from build123d import *
from build123d.topology import SkipClean

# Parameters (mm, degrees)
SKETCH1_R            = 1.5
BOSS_EXTRUDE1_DEPTH  = 2
BOSS_EXTRUDE2_START  = 3
SKETCH2_R            = 2.5
SKETCH2_R_2          = 1.5
BOSS_EXTRUDE2_DEPTH  = 3
CUT_EXTRUDE1_REACH   = 126.021
SKETCH3_R            = 2.5
LPATTERN1_COUNT      = 3
LPATTERN1_PITCH      = 40.75
LPATTERN1_COUNT_DIR2 = 3
LPATTERN1_PITCH_DIR2 = 10
SKETCH4_W            = 2
SKETCH4_H            = 29.25
BOSS_EXTRUDE3_DEPTH  = 2


with BuildPart() as part:
    # Sketch1 → Boss-Extrude1 (new body)
    with BuildSketch(Plane(origin=(0, 0, 0), x_dir=(1, 0, 0), z_dir=(0, 1, 0))):
        Polygon((-112.25, 0), (0, 0), (0, 33.5), (-16, 33.5), (-16, 52.5), (-112.25, 52.5), align=None)
        with Locations(Location((-47.25, 49, 0), (0, 0, 270))):
            Circle(SKETCH1_R, mode=Mode.SUBTRACT)
        with Locations(Location((-108.75, 37.5, 0), (0, 0, 270))):
            Circle(SKETCH1_R, mode=Mode.SUBTRACT)
    extrude(amount=BOSS_EXTRUDE1_DEPTH)

    # Sketch2 → Boss-Extrude2 (add)
    with SkipClean():  # the faces are left unmerged after this step: merging them gives an invalid solid
        with BuildSketch(Plane(origin=(0, 0, 0), x_dir=(-1, 0, 0), z_dir=(0, -1, 0)).offset(BOSS_EXTRUDE2_START)):
            with Locations(Location((108.75, 37.5, 0), (0, 0, 90))):
                Circle(SKETCH2_R)
            with Locations(Location((108.75, 37.5, 0), (0, 0, 90))):
                Circle(SKETCH2_R_2, mode=Mode.SUBTRACT)
        extrude(amount=-BOSS_EXTRUDE2_DEPTH)

    # Sketch3 → Cut-Extrude1 (cut, up to next)
    with BuildSketch(Plane(origin=(0, 2, 0), x_dir=(1, 0, 0), z_dir=(0, 1, 0)), mode=Mode.PRIVATE) as cut_extrude1_sk1:
        with Locations(Location((-3.75, 26.75, 0), (0, 0, 270))):
            Circle(SKETCH3_R)
    cut_extrude1_tool1 = extrude(cut_extrude1_sk1.sketch, amount=-CUT_EXTRUDE1_REACH, mode=Mode.PRIVATE) & part.part
    # Sketch3 → Cut-Extrude1 (cut, up to next)
    with BuildSketch(Plane(origin=(0, 2, 0), x_dir=(1, 0, 0), z_dir=(0, 1, 0)), mode=Mode.PRIVATE) as cut_extrude1_sk2:
        with BuildLine():
            Line((-37.25, 29.25), (-11.25, 29.25))
            ThreePointArc((-11.25, 29.25), (-8.75, 26.75), (-11.25, 24.25))
            Line((-11.25, 24.25), (-37.25, 24.25))
            ThreePointArc((-37.25, 24.25), (-39.75, 26.75), (-37.25, 29.25))
        make_face()
    cut_extrude1_tool2 = extrude(cut_extrude1_sk2.sketch, amount=-CUT_EXTRUDE1_REACH, mode=Mode.PRIVATE) & part.part
    cut_extrude1_1 = cut_extrude1_tool1.solids().sort_by_distance((-3.75, 2, -26.75))[0]
    add(cut_extrude1_1, mode=Mode.SUBTRACT)
    cut_extrude1_2 = cut_extrude1_tool2.solids().sort_by_distance((-24.25, 2, -26.75))[0]
    add(cut_extrude1_2, mode=Mode.SUBTRACT)
    cut_extrude1 = cut_extrude1_1 + cut_extrude1_2  # Cut-Extrude1 as one shape, for the pattern or mirror that repeats it

    # LPattern1: Cut-Extrude1 3 × 3
    with SkipClean():  # the faces are left unmerged after this step: merging them gives an invalid solid
        with Locations(*[(-i * LPATTERN1_PITCH, 0, j * LPATTERN1_PITCH_DIR2) for i in range(LPATTERN1_COUNT) for j in range(LPATTERN1_COUNT_DIR2) if (i, j) != (0, 0)]):
            add(cut_extrude1, mode=Mode.SUBTRACT)

    # Sketch4 → Boss-Extrude3 (add)
    with SkipClean():  # the faces are left unmerged after this step: merging them gives an invalid solid
        with BuildSketch(Plane(origin=(0, 2, 0), x_dir=(1, 0, 0), z_dir=(0, 1, 0))):
            with Locations((-111.25, 14.625)):
                Rectangle(SKETCH4_W, SKETCH4_H)
        extrude(amount=-BOSS_EXTRUDE3_DEPTH)


solid = part.part
Can you work these out from the model? Positions are in its coordinate system, mm. A direction names the side the tool comes from. Round coordinates to 2 decimals unless told otherwise and drop trailing zeros. Write each loop counter-clockwise with the first axis right and the second up, starting at its lowest first coordinate (ties: lowest second). Pieces come first, ordered by that corner, then holes. Notation, with made-up numbers: (84, 80.5) -> (88, 80.5) arc R20 cw to (88, 113.5) -> close; hole circle Ø6 at (83.25, -1). An arc over 180 degrees is marked (long way). One line per question, with ' | ' between items. Start each with the question number.
1) Suppose I cut it at B-B on z = -26.75. Write out the boundary of the cut face in (x, y).
2) I'm going to push flat-ended pins straight in: P1, Ø6.5, axis at x = -44.5, z = -26.75, coming from the -Y side; P2, Ø2, axis at y = -2, z = -12, coming from the +X side; P3, Ø2, axis at y = 1, z = -43, coming from the +X side. Where does each tip first touch, or does it pass through?
3) Suppose I cut it at C-C on y = -1.35. Write out the boundary of the cut face in (x, z), then the cut area to 3 significant figures.
4) Suppose I cut it at A-A on x = -85.25. Write out the boundary of the cut face in (y, z), then the cut area to 3 significant figures.
5) On a 3-axis mill with a long thin cutter (end or side, diameter ignored), from which of +Z, -Z, +X, -X, +Y, -Y can I reach the whole of each face in a straight line? I mean faces 1 (the cylindrical face through (-90.25, 1.01, -26.8)), 2 (the flat face through (0, 1, -17)). Say none if no direction works.
6) If we mould it in two halves opening along X, with no side actions, what happens to faces 3 (the flat face through (-102, 1, -19.25)), 4 (the flat face through (-65, 1, -29.25)), 5 (the flat face through (-112.25, 1, -27)), 6 (the flat face through (-110, -3, -39))? For each: released by +X, released by -X, zero draft, split by the parting line, or undercut.
7) I need wall thicknesses on line 1 (Z direction, x = -20, y = 1.05); line 2 (X direction, y = 0.5, z = -49); line 3 (Y direction, x = -69.5, z = -42.5). Which ranges of each line are inside material? Lowest first, please. Write a range as [from, to].
8) Suppose I cut it at D-D on z = -17. Write out the boundary of the cut face in (x, y).
Return value:
1) outline: (-112.25, 0) -> (-110.25, 0) -> (-110.25, 2) -> (-112.25, 2) -> close; (-90.25, 0) -> (-87.75, 0) -> (-87.75, 2) -> (-90.25, 2) -> close; (-82.75, 0) -> (-80.5, 0) -> (-80.5, 2) -> (-82.75, 2) -> close; (-49.5, 0) -> (-47, 0) -> (-47, 2) -> (-49.5, 2) -> close; (-42, 0) -> (-39.75, 0) -> (-39.75, 2) -> (-42, 2) -> close; (-8.75, 0) -> (-6.25, 0) -> (-6.25, 2) -> (-8.75, 2) -> close; (-1.25, 0) -> (0, 0) -> (0, 2) -> (-1.25, 2) -> close
2) P1: stops at y = 0 | P2: passes through | P3: stops at x = -16
3) outline: circle Ø5 at (-108.75, -37.5); hole circle Ø3 at (-108.75, -37.5) | area: 12.6 mm2
4) outline: (0, -52.5) -> (2, -52.5) -> (2, -29.25) -> (0, -29.25) -> close; (0, -24.25) -> (2, -24.25) -> (2, -19.25) -> (0, -19.25) -> close; (0, -14.25) -> (2, -14.25) -> (2, -9.25) -> (0, -9.25) -> close; (0, -4.25) -> (2, -4.25) -> (2, 0) -> (0, 0) -> close | area: 75.0 mm2
5) face 1: +Y, -Y | face 2: +Z, -Z, +X, +Y, -Y
6) face 3: undercut | face 4: undercut | face 5: released by -X | face 6: zero draft
7) line 1: z = [-52.5, -29.25], [-24.25, -19.25], [-14.25, -9.25], [-4.25, 0] | line 2: x = [-112.25, -48.75], [-45.75, -16] | line 3: y = [0, 2]
8) outline: (-112.25, 0) -> (-110.25, 0) -> (-110.25, 2) -> (-112.25, 2) -> close; (-90.26, 0) -> (-87.74, 0) -> (-87.74, 2) -> (-90.26, 2) -> close; (-82.76, 0) -> (-80.49, 0) -> (-80.49, 2) -> (-82.76, 2) -> close; (-49.51, 0) -> (-46.99, 0) -> (-46.99, 2) -> (-49.51, 2) -> close; (-42.01, 0) -> (-39.74, 0) -> (-39.74, 2) -> (-42.01, 2) -> close; (-8.76, 0) -> (-6.24, 0) -> (-6.24, 2) -> (-8.76, 2) -> close; (-1.26, 0) -> (0, 0) -> (0, 2) -> (-1.26, 2) -> close
